Read the model definition and answer for the solid it produces. Units are mm, in the model's axes. A direction names the side the tool comes from. Coordinates: 2 decimals unless noted, no trailing zeros. Order: outer loops, then holes, each group sorted by start corner. A loop starts at its lowest first (then second) coordinate and runs counter-clockwise, first axis right, second up. Notation, with made-up numbers: (56.5, 72.25) - (70.5, 72.25) arc R29 ccw to (70.5, 104.25) - close; hole circle Ø11 at (-33.5, -35.75). An arc over 180 degrees is marked (long way). Use one line per item in the form item = value.
```python
from build123d import *

# Parameters (mm, degrees)
F0_W     = 127
F0_H     = 25.4
F1_DEPTH = 5
F2_W     = 160
F2_H     = 25.4
F3_DEPTH = 5
F4_R     = 4.9784
F5_DEPTH = 40


with BuildPart() as f1:
    # F0 (on Front) → F1 (new body)
    with BuildSketch(Plane.XZ):
        Rectangle(F0_W, F0_H)
    extrude(amount=-F1_DEPTH)

    # F2 (on Front) → F3 (join, through all)
    with BuildSketch(Plane.XZ):
        with Locations((-143.5, 0)):
            Rectangle(F2_W, F2_H)
    extrude(amount=-F3_DEPTH)

    # F4 (on face) → F5 (join)
    with BuildSketch(Plane(origin=(0, 5, 0), x_dir=(-1, 0, 0), z_dir=(0, 1, 0))):
        with Locations((-52.375, 0)):
            Circle(F4_R)
        with Locations((52.375, 0)):
            Circle(F4_R)
        with Locations((201.934084, 0)):
            Circle(F4_R)
    extrude(amount=-F5_DEPTH)


solid = f1.part
```
(1) Straight lines are drawn through the part: L1, parallel to X at y = -7, z = -0.5; L2, parallel to Y at x = 9, z = 5.75; L3, parallel to X at y = -20.5, z = 4.5. For each, find the intervals that lie inside material, in ascending order.
Answer list:
L1 = -206.89 to -196.98, -57.33 to -47.42, 47.42 to 57.33
L2 = 0 to 5
L3 = -204.06 to -199.8, -54.5 to -50.25, 50.25 to 54.5
(2) The mould has two halves that part along X. Classify faces 3 (the cylindrical face through (-47.4, -17.3, 0.2)), 4 (the cylindrical face through (57.35, -17.26, 0.22)), 5 (the flat face through (-202, -35, 0)), 6 (the flat face through (-223.5, 2, 0)): +X half, -X half, draft (parallel to the pull), parting line (faces both ways), or undercut.
Answer list:
face_3 = undercut
face_4 = undercut
face_5 = draft
face_6 = -X half
(3) Section A-A, the plane z = 0 is taken. Write down the section's boundary in (x, y).
Answer list:
outline = (-223.5, 0) - (-206.91, 0) - (-206.91, -35) - (-196.96, -35) - (-196.96, 0) - (-57.35, 0) - (-57.35, -35) - (-47.4, -35) - (-47.4, 0) - (47.4, 0) - (47.4, -35) - (57.35, -35) - (57.35, 0) - (63.5, 0) - (63.5, 5) - (-223.5, 5) - close
(4) Section B-B, the plane y = -21 is taken. Write down the section's boundary in (x, z) (3 decimals).
Answer list:
outline = circle Ø9.957 at (-201.934, 0); circle Ø9.957 at (-52.375, 0); circle Ø9.957 at (52.375, 0)
(5) Given pin 1 Ø1 at (x, y) = (-72, -1.5) entering from +Z; pin 2 Ø3 at (x, z) = (-91.5, -9) entering from -Y; pin 3 Ø5 at (y, z) = (-21.5, 4.5) entering from +X, each flat-ended and moving along its own axis, determine where each tip first touches the part or whether it passes through.
Answer list:
pin_1 = through
pin_2 = 0
pin_3 = 56.93
(6) Which of the six approach directions +Z, -Z, +X, -X, +Y, -Y give full straight-line access (tool end or side, diameter ignored) to faces 1 (the flat face through (-82, 2, -12.7)), 2 (the cylindrical face through (-206.53, -17.26, -1.91))?
Answer list:
face_1 = -Z, +X, -X, +Y, -Y
face_2 = -Y
(7) Section C-C, the plane x = 19 is taken. Write down the section's boundary in (y, z), then the cut area to 3 significant figures.
Answer list:
outline = (0, -12.7) - (5, -12.7) - (5, 12.7) - (0, 12.7) - close
area = 127 mm2
